Can you work these out from the model? Positions are in its coordinate system, mm. Round coordinates to 2 decimals unless told otherwise and drop trailing zeros. Write each loop counter-clockwise with the first axis right and the second up, starting at its lowest first coordinate (ties: lowest second). Pieces come first, ordered by that corner, then holes. Notation, with made-up numbers: M 61.5,73 L 75.5,73 A10 ccw 75.5,83 Z; hole C 35.5,39.5 d5. An arc over 180 degrees is marked long. Answer as a JSON object with one key per item and string values. Group by question number.
1) Suppose I cut it at B-B, the plane y = 8. Write out the boundary of the cut face in (x, z).
2) Suppose I cut it at D-D, the plane x = 21. Write out the boundary of the cut face in (y, z).
3) Suppose I cut it at C-C, the plane z = 42.5. Write out the boundary of the cut face in (x, y).
4) Please list where these lines run through material, in increasing order: L1, parallel to Z at x = 74, y = 2.75; L2, parallel to X at y = 3.5, z = -42.5; L3, parallel to X at y = 2, z = 85. Write a range as [from, to].
5) Suppose I cut it at A-A, the plane z = 85. Write out the boundary of the cut face in (x, y), and give its area (3 significant figures).
6) I'm going to push flat-ended pins straight in: pin 1 Ø4 at (x, z) = (-73.61, 42.5) entering from +Y; pin 2 Ø3 at (x, y) = (74.5, 8.5) entering from -Z; pin 3 Ø6 at (y, z) = (8.5, 68.5) entering from +X; pin 4 Ø8.5 at (x, z) = (73.61, 42.5) entering from +Y. Where does each tip first touch, or does it pass through?
from build123d import *

# Parameters (mm, degrees)
SKETCH1_R                                        = 100
BOSS_EXTRUDE1_DEPTH                              = 10
CSK_FOR_1_4_FLAT_HEAD_MACHINE_SCREW1_D           = 6.5278
CSK_FOR_1_4_FLAT_HEAD_MACHINE_SCREW1_DEPTH       = 10
CSK_FOR_1_4_FLAT_HEAD_MACHINE_SCREW1_CSINK_D     = 12.8778
CSK_FOR_1_4_FLAT_HEAD_MACHINE_SCREW1_CSINK_ANGLE = 82
CSK_FOR_1_4_FLAT_HEAD_MACHINE_SCREW1_TIP         = 1.961148974


with BuildPart() as part:
    # Sketch1 → Boss-Extrude1 (new body)
    with BuildSketch(Plane(origin=(0, 0, 0), x_dir=(1, 0, 0), z_dir=(0, 1, 0))):
        with Locations(Location((0, 0, 0), (0, 0, 270))):
            Circle(SKETCH1_R)
    extrude(amount=BOSS_EXTRUDE1_DEPTH)

    # CSK for 1/4 Flat Head Machine Screw1
    with Locations(Plane(origin=(0, 10, 0), x_dir=(1, 0, 0), z_dir=(0, 1, 0))):
        with Locations((-73.612159322, 42.5), (0, 85), (73.612159322, 42.5), (73.612159322, -42.5), (0, -85), (-73.612159322, -42.5)):
            CounterSinkHole(CSK_FOR_1_4_FLAT_HEAD_MACHINE_SCREW1_D / 2, CSK_FOR_1_4_FLAT_HEAD_MACHINE_SCREW1_CSINK_D / 2, depth=CSK_FOR_1_4_FLAT_HEAD_MACHINE_SCREW1_DEPTH, counter_sink_angle=CSK_FOR_1_4_FLAT_HEAD_MACHINE_SCREW1_CSINK_ANGLE)
            with Locations((0, 0, -(CSK_FOR_1_4_FLAT_HEAD_MACHINE_SCREW1_DEPTH + CSK_FOR_1_4_FLAT_HEAD_MACHINE_SCREW1_TIP / 2))):  # 118° drill point
                Cone(0, CSK_FOR_1_4_FLAT_HEAD_MACHINE_SCREW1_D / 2, CSK_FOR_1_4_FLAT_HEAD_MACHINE_SCREW1_TIP, mode=Mode.SUBTRACT)


solid = part.part
Results:
{
 "1": {"outline": "C 0,0 d200; hole C -73.61,-42.5 d9.4; hole C -73.61,42.5 d9.4; hole C 0,-85 d9.4; hole C 0,85 d9.4; hole C 73.61,-42.5 d9.4; hole C 73.61,42.5 d9.4"},
 "2": {"outline": "M 0,-97.77 L 10,-97.77 L 10,97.77 L 0,97.77 Z"},
 "3": {"outline": "M -90.52,0 L -76.88,0 L -76.88,6.35 L -80.05,10 L -90.52,10 Z; M -70.35,0 L 70.35,0 L 70.35,6.35 L 67.17,10 L -67.17,10 L -70.35,6.35 Z; M 76.88,0 L 90.52,0 L 90.52,10 L 80.05,10 L 76.88,6.35 Z"},
 "4": {"L1": "[-67.26, -45.74], [-39.26, 39.26], [45.74, 67.26]", "L2": "[-90.52, -76.88], [-70.35, 70.35], [76.88, 90.52]", "L3": "[-52.68, -3.26], [3.26, 52.68]"},
 "5": {"outline": "M -52.68,0 L -3.26,0 L -3.26,6.35 L -6.44,10 L -52.68,10 Z; M 3.26,0 L 52.68,0 L 52.68,10 L 6.44,10 L 3.26,6.35 Z", "area": "977 mm^2"},
 "6": {"pin 1": "through", "pin 2": "z = -68.34", "pin 3": "x = 75.56", "pin 4": "y = 7.48"}
}
